Here's the drawing with two shaded views (mm, measured from the low corner). I have some questions. A direction names the side the tool comes from. Coordinates: 2 decimals unless noted, no trailing zeros. Loops run counter-clockwise (first coordinate to the right, second up) from the corner with the lowest first, then second, coordinate; pieces in that order, holes last. Notation, with made-up numbers: (-10.75, -40) -> (12.25, -40) arc R26 ccw to (12.25, -17) -> close; hole circle Ø11 at (-31.5, 22.25). An arc over 180 degrees is marked (long way). Answer as a JSON object with one key per item and string values. Group by question number.
Q1. I want a section at C-C on y = 4. Write out the boundary of the cut face in (x, z).
Q2. On a 3-axis mill with a long thin cutter (end or side, diameter ignored), from which of +Z, -Z, +X, -X, +Y, -Y can I reach the whole of each face in a straight line? I mean the marked faces 1 and 2. Say none if no direction works.
Q3. I'm going to push flat-ended pins straight in: pin 1 (3 mm diameter, centred on x = 26.5, y = 4.5, fed in from -Z) (1 decimal); pin 2 (8 mm diameter, centred on x = 23, y = 15.5, fed in from +Z); pin 3 (12.5 mm diameter, centred on x = 12, z = 9, fed in from +Y); pin 4 (4 mm diameter, centred on x = 5, y = 3, fed in from -Z) (3 decimals). Where does each tip first touch, or does it pass through?
Q4. I want a section at B-B on x = 27. Write out the boundary of the cut face in (y, z).
Q5. I need wall thicknesses on line 1 (Y direction, x = 9, z = 24.5); line 2 (Y direction, x = 24.5, z = 2.5); line 3 (X direction, y = 5.25, z = 15). Which ranges of each line are inside material? Lowest first, please.
Q6. Thinking about a two-plate mould opening in Z: for the marked faces 3, 4 and 5, which applies, released by +Z, released by -Z, zero draft, split by the parting line, or undercut?
Q7. I want a section at A-A on z = 3.5. Write out the boundary of the cut face in (x, y).
Q8. I want a section at D-D on y = 8.25. Write out the boundary of the cut face in (x, z), then the cut area to 3 significant figures.
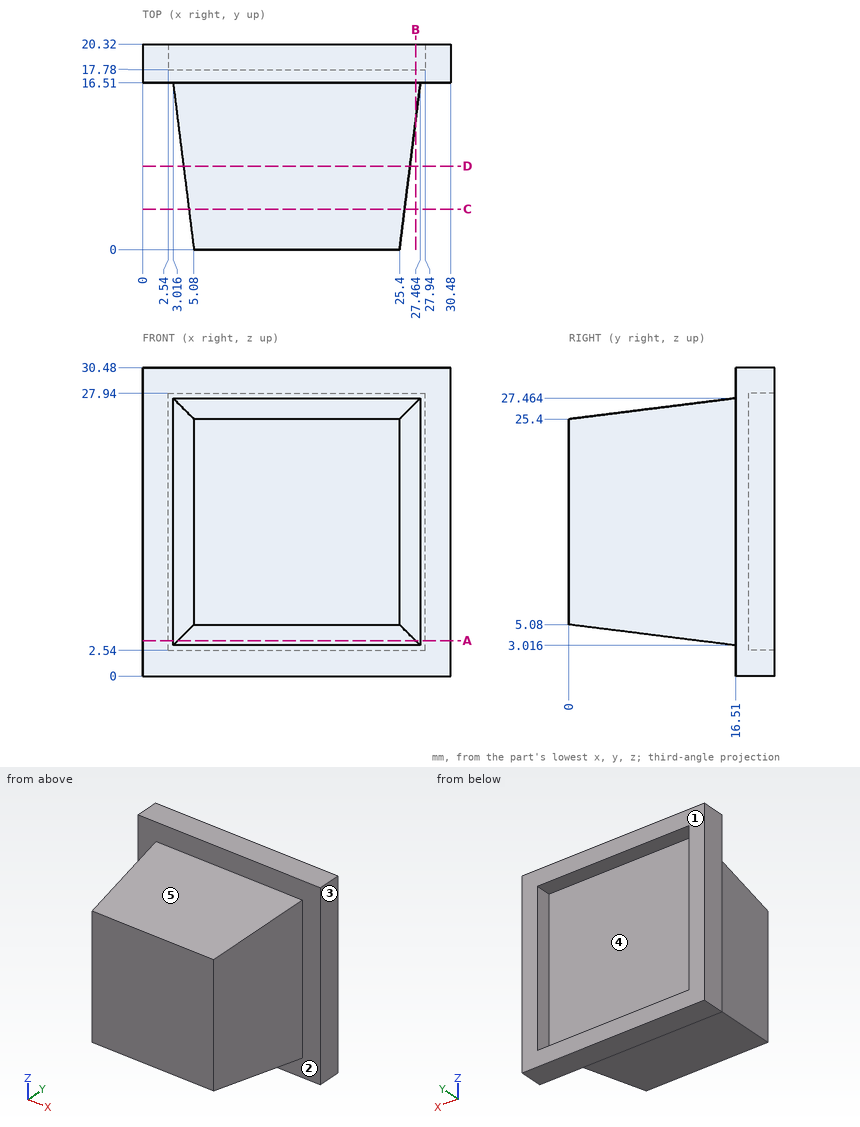
Result set:
{
 "1": {"outline": "(4.58, 4.58) -> (25.9, 4.58) -> (25.9, 25.9) -> (4.58, 25.9) -> close"},
 "2": {"face 1": "+Z, -Z, +X, -X, +Y", "face 2": "-Y"},
 "3": {"pin 1": "stops at z = 4.3", "pin 2": "stops at z = 30.48", "pin 3": "stops at y = 17.78", "pin 4": "stops at z = 4.455"},
 "4": {"outline": "(12.8, 3.48) -> (16.51, 3.02) -> (16.51, 0) -> (20.32, 0) -> (20.32, 2.54) -> (17.78, 2.54) -> (17.78, 27.94) -> (20.32, 27.94) -> (20.32, 30.48) -> (16.51, 30.48) -> (16.51, 27.46) -> (12.8, 27) -> close"},
 "5": {"line 1": "y = 0 to 17.78", "line 2": "y = 16.51 to 20.32", "line 3": "x = 4.42 to 26.06"},
 "6": {"face 3": "zero draft", "face 4": "undercut", "face 5": "released by +Z"},
 "7": {"outline": "(0, 16.51) -> (3.02, 16.51) -> (3.5, 12.64) -> (26.98, 12.64) -> (27.46, 16.51) -> (30.48, 16.51) -> (30.48, 20.32) -> (27.94, 20.32) -> (27.94, 17.78) -> (2.54, 17.78) -> (2.54, 20.32) -> (0, 20.32) -> close"},
 "8": {"outline": "(4.05, 4.05) -> (26.43, 4.05) -> (26.43, 26.43) -> (4.05, 26.43) -> close", "area": "501 mm²"}
}
